Verification items for the finished model (mm, model axes). Face numbers are marked on the shaded views. Round coordinates to 2 decimals unless told otherwise and drop trailing zeros. Write each loop counter-clockwise with the first axis right and the second up, starting at its lowest first coordinate (ties: lowest second). Pieces come first, ordered by that corner, then holes. Notation, with made-up numbers: M 47.5,59.5 L 77.5,59.5 A18 ccw 77.5,84.5 Z; hole C 57.5,18.5 d10. An arc over 180 degrees is marked long. One line per question, with ' | ' between items. Start each with the question number.
Q1. Release check for a two-part mould opening along X. For the marked faces 1 and 2 record: released by +X, released by -X, zero draft, split by the parting line, or undercut.
Q2. Gauge pin test, flat ends, axial feed: pin 1 (2 mm diameter, centred on x = -36.5, y = -1.5, fed in from +Z); pin 2 (2 mm diameter, centred on y = -7.5, z = 227, fed in from -X); pin 3 (1.5 mm diameter, centred on x = -73, z = 204.5, fed in from +Y); pin 4 (2 mm diameter, centred on y = -2.5, z = 186.5, fed in from +X). Record the tip position at first contact, or that the pin passes through.
Q3. Cross-section at C-C (z = 204.5). Record the boundary of the cut face in (x, y).
Q4. Cross-section at D-D (x = 1). Record the boundary of the cut face in (y, z).
Q5. Thickness scan on line 1 along X through (y, z) = (-1.5, 200); line 2 along X through (y, z) = (-4, 196); line 3 along Z through (x, y) = (-16, -10.75). Record the ranges inside material, lowest first. Write a range as from..to.
Q6. Cross-section at A-A (y = -2). Record the boundary of the cut face in (x, z).
Q7. Cross-section at B-B (z = 194). Record the boundary of the cut face in (x, y), then the cut area to 3 significant figures.
from build123d import *

# Parameters (mm, degrees)
F0_R     = 27.05
F1_DEPTH = 12


with BuildPart() as f1:
    # F0 (on Front) → F1 (new body)
    with BuildSketch(Plane.XZ):
        with BuildLine():
            Line((-66.333731852, 225.8735977012), (-88.4299040636, 207.3600747496))
            ThreePointArc((-88.4299040636, 207.3600747496), (-83.0164485889, 209.5079378807), (-77.2292867797, 208.8540461453))
            ThreePointArc((-77.2292867797, 208.8540461453), (-72.9336199483, 218.1013786467), (-66.333731852, 225.8735977012))
        make_face()
        with BuildLine():
            ThreePointArc((-88.4299040636, 207.3600747496), (-92.1069823157, 203.0905059798), (-93.4299040636, 197.6132804047))
            ThreePointArc((-93.4299040636, 197.6132804047), (-92.1069823157, 192.1360548297), (-88.4299040636, 187.8664860599))
            ThreePointArc((-88.4299040636, 187.8664860599), (-83.0164485889, 185.7186229288), (-77.2292867797, 186.3725146642))
            ThreePointArc((-77.2292867797, 186.3725146642), (-78.0429869708, 189.4512293681), (-78.5960579098, 192.5872626533))
            ThreePointArc((-78.5960579098, 192.5872626533), (-85.1299040636, 197.6132804047), (-78.5960579098, 202.6392981562))
            ThreePointArc((-78.5960579098, 202.6392981562), (-78.0429869708, 205.7753314414), (-77.2292867797, 208.8540461453))
            ThreePointArc((-77.2292867797, 208.8540461453), (-83.0164485889, 209.5079378807), (-88.4299040636, 207.3600747496))
        make_face()
        with BuildLine():
            ThreePointArc((-64.3060042971, 167.6540090873), (-53.2900757844, 161.6796449773), (-40.9299040636, 159.6132804047))
            ThreePointArc((-40.9299040636, 159.6132804047), (-28.5697323428, 161.6796449773), (-17.5538038301, 167.6540090873))
            Line((-17.5538038301, 167.6540090873), (-15.5260762752, 169.3529631083))
            ThreePointArc((-15.5260762752, 169.3529631083), (-8.9261881789, 177.1251821628), (-4.6305213476, 186.3725146642))
            ThreePointArc((-4.6305213476, 186.3725146642), (-3.8168211564, 189.4512293681), (-3.2637502175, 192.5872626533))
            ThreePointArc((-3.2637502175, 192.5872626533), (-7.1299040636, 197.6132804047), (-3.2637502175, 202.6392981562))
            ThreePointArc((-3.2637502175, 202.6392981562), (-3.8168211564, 205.7753314414), (-4.6305213476, 208.8540461453))
            ThreePointArc((-4.6305213476, 208.8540461453), (-8.9261881789, 218.1013786467), (-15.5260762752, 225.8735977012))
            Line((-15.5260762752, 225.8735977012), (-17.5538038301, 227.5725517222))
            ThreePointArc((-17.5538038301, 227.5725517222), (-28.5697323428, 233.5469158322), (-40.9299040636, 235.6132804047))
            ThreePointArc((-40.9299040636, 235.6132804047), (-53.2900757844, 233.5469158322), (-64.3060042971, 227.5725517222))
            Line((-64.3060042971, 227.5725517222), (-66.333731852, 225.8735977012))
            ThreePointArc((-66.333731852, 225.8735977012), (-72.9336199483, 218.1013786467), (-77.2292867797, 208.8540461453))
            ThreePointArc((-77.2292867797, 208.8540461453), (-78.0429869708, 205.7753314414), (-78.5960579098, 202.6392981562))
            ThreePointArc((-78.5960579098, 202.6392981562), (-75.8082539087, 200.783769326), (-74.7299040636, 197.6132804047))
            ThreePointArc((-74.7299040636, 197.6132804047), (-75.8082539087, 194.4427914835), (-78.5960579098, 192.5872626533))
            ThreePointArc((-78.5960579098, 192.5872626533), (-78.0429869708, 189.4512293681), (-77.2292867797, 186.3725146642))
            ThreePointArc((-77.2292867797, 186.3725146642), (-72.9336199483, 177.1251821628), (-66.333731852, 169.3529631083))
            Line((-66.333731852, 169.3529631083), (-64.3060042971, 167.6540090873))
        make_face()
        with Locations((-40.9299040636, 197.6132804047)):
            Circle(F0_R, mode=Mode.SUBTRACT)
        with BuildLine():
            ThreePointArc((-77.2292867797, 186.3725146642), (-83.0164485889, 185.7186229288), (-88.4299040636, 187.8664860599))
            Line((-88.4299040636, 187.8664860599), (-66.333731852, 169.3529631083))
            ThreePointArc((-66.333731852, 169.3529631083), (-72.9336199483, 177.1251821628), (-77.2292867797, 186.3725146642))
        make_face()
        with BuildLine():
            ThreePointArc((-4.6305213476, 186.3725146642), (-8.9261881789, 177.1251821628), (-15.5260762752, 169.3529631083))
            Line((-15.5260762752, 169.3529631083), (6.5700959364, 187.8664860599))
            ThreePointArc((6.5700959364, 187.8664860599), (1.1566404616, 185.7186229288), (-4.6305213476, 186.3725146642))
        make_face()
        with BuildLine():
            ThreePointArc((-4.6305213476, 208.8540461453), (1.1566404616, 209.5079378807), (6.5700959364, 207.3600747496))
            Line((6.5700959364, 207.3600747496), (-15.5260762752, 225.8735977012))
            ThreePointArc((-15.5260762752, 225.8735977012), (-8.9261881789, 218.1013786467), (-4.6305213476, 208.8540461453))
        make_face()
        with BuildLine():
            ThreePointArc((6.5700959364, 187.8664860599), (10.2471741992, 192.1360548507), (11.5700959364, 197.613280452))
            ThreePointArc((11.5700959364, 197.613280452), (10.2471741776, 203.0905060008), (6.5700959364, 207.3600747496))
            ThreePointArc((6.5700959364, 207.3600747496), (1.1566404616, 209.5079378807), (-4.6305213476, 208.8540461453))
            ThreePointArc((-4.6305213476, 208.8540461453), (-3.8168211564, 205.7753314414), (-3.2637502175, 202.6392981562))
            ThreePointArc((-3.2637502175, 202.6392981562), (1.2405848577, 201.7349305597), (3.2700959364, 197.6132804047))
            ThreePointArc((3.2700959364, 197.6132804047), (1.2405848577, 193.4916302498), (-3.2637502175, 192.5872626533))
            ThreePointArc((-3.2637502175, 192.5872626533), (-3.8168211564, 189.4512293681), (-4.6305213476, 186.3725146642))
            ThreePointArc((-4.6305213476, 186.3725146642), (1.1566404616, 185.7186229288), (6.5700959364, 187.8664860599))
        make_face()
    extrude(amount=F1_DEPTH)


solid = f1.part
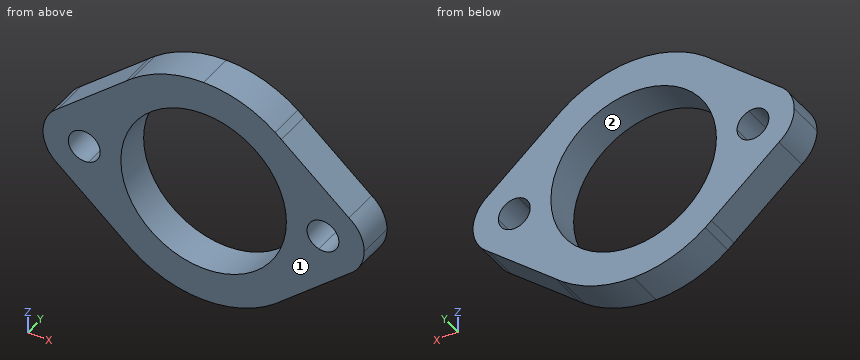
Determined:
1) face 1: zero draft | face 2: undercut
2) pin 1: stops at z = 235.46 | pin 2: stops at x = -66.18 | pin 3: stops at y = 0 | pin 4: stops at x = 6.13
3) outline: M -91.26,-12 L -67.09,-12 L -67.09,0 L -91.26,0 Z; M -14.77,-12 L 9.4,-12 L 9.4,0 L -14.77,0 Z
4) outline: M -12,183.2 L 0,183.2 L 0,193.32 L -12,193.32 Z; M -12,201.91 L 0,201.91 L 0,212.03 L -12,212.03 Z
5) line 1: x = -93.19..-84.55, -75.31..-67.87, -13.99..-6.55, 2.69..11.33 | line 2: x = -93.32..-84.87, -74.99..-67.93, -13.93..-6.87, 3.01..11.46 | line 3: z = 168.96..187.12, 208.11..226.27
6) outline: M -88.43,187.87 L -64.31,167.65 A38 ccw -17.55,167.65 L 6.57,187.87 A12 ccw 6.57,207.36 L -17.55,227.57 A38 ccw -64.31,227.57 L -88.43,207.36 A12 ccw Z; hole C -79.93,197.61 d10.4; hole C -40.93,197.61 d54.1; hole C -1.93,197.61 d10.4
7) outline: M -92.87,-12 L -83.67,-12 L -83.67,0 L -92.87,0 Z; M -76.19,-12 L -67.74,-12 L -67.74,0 L -76.19,0 Z; M -14.12,-12 L -5.67,-12 L -5.67,0 L -14.12,0 Z; M 1.81,-12 L 11.01,-12 L 11.01,0 L 1.81,0 Z | area: 424 mm²
